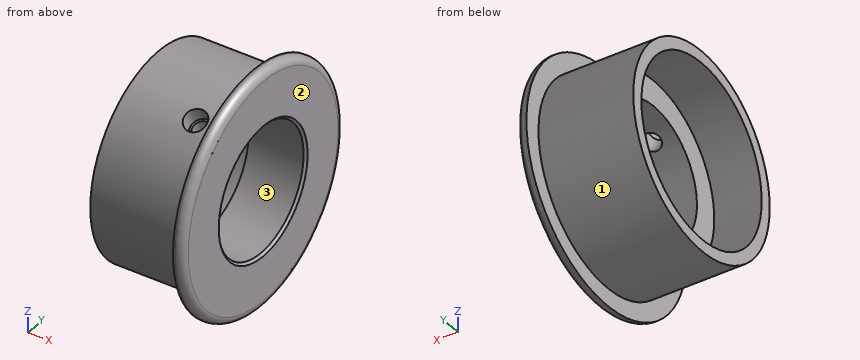
from build123d import *

# Parameters (mm, degrees)
SKETCH144_R     = 2.25
HOLE050_DEPTH   = 40.84516
SKETCH145_R     = 2.8
POCKET198_DEPTH = 4.5
CHAMFER002_SIZE = 0.6


with BuildPart() as part:
    # Sketch143 → Revolution004 (revolve)
    with BuildSketch(Plane.XZ):
        with BuildLine():
            Line((0, 25.4), (0, 29.9))
            Line((0, 29.9), (0.5, 29.9))
            ThreePointArc((2.5, 27.9), (1.914214, 29.314214), (0.5, 29.9))
            Line((2.5, 27.9), (2.5, 15.95))
            Line((2.5, 15.95), (-12, 15.95))
            Line((-12, 15.95), (-12, 22.4))
            Line((-12, 22.4), (-24, 22.4))
            Line((-24, 22.4), (-24, 25.4))
            Line((-24, 25.4), (0, 25.4))
        make_face()
    revolve(axis=Axis((0, 0, 0), (1, 0, 0)))

    # Sketch144 (on DatumPlane) → Hole050 (cut, through all)
    with BuildSketch(Plane(origin=(-6, 0, 0), x_dir=(1, 0, 0), z_dir=(0, 0.5, -0.866025))):
        Circle(SKETCH144_R)
    extrude(amount=-HOLE050_DEPTH, mode=Mode.SUBTRACT)

    # Sketch145 (on DatumPlane) → Pocket198 (cut)
    with BuildSketch(Plane(origin=(-6, -12.7, 21.997045), x_dir=(-1, 0, 0), z_dir=(0, -0.5, 0.866025))):
        Circle(SKETCH145_R)
    extrude(amount=-POCKET198_DEPTH, mode=Mode.SUBTRACT)

    # Chamfer002
    chamfer002_edges = [part.edges().sort_by_distance(p)[0] for p in [
        (2.5, 0, -15.95),
    ]]
    chamfer(chamfer002_edges, length=CHAMFER002_SIZE)


with BuildPart() as part_1:
    # Body022029 placement: moved
    add(part.part.moved(Location((194, 0, 835))))


solid = part_1.part
Model file for the job. Use its own axes, mm. Face numbers are marked on the shaded views. Give positions to 0.01 mm unless a question says otherwise; leave off trailing zeros. Order: outer loops, then holes, each group sorted by start corner. A loop starts at its lowest first (then second) coordinate and runs counter-clockwise, first axis right, second up. Notation, with made-up numbers: (86, 7) -> (92, 7) arc R28 ccw to (92, 30) -> close; hole circle Ø6 at (-14.75, 20). An arc over 180 degrees is marked (long way). Use CSV: the item, a comma, the result in double quotes.
1. Drop flat-ended pins along their axis: pin 1 (6 mm diameter, centred on x = 190, y = -12, fed in from -Z); pin 2 (8 mm diameter, centred on x = 192.5, y = -11.5, fed in from +Z); pin 3 (4 mm diameter, centred on x = 185.5, y = 16.5, fed in from +Z). Give the stop position or say it passes through.
Outcome:
pin 1,"z = 811.25"
pin 2,"z = 863.87"
pin 3,"z = 855.85"
2. Mould opens along Z. For the marked faces 1, 2 and 3 say: +Z half, -Z half, draft (parallel to the pull), parting line (faces both ways), or undercut.
Outcome:
face 1,"parting line"
face 2,"draft"
face 3,"undercut"
3. Band-saw the part on B-B, the plane y = 0. Give the cut face in (x, z).
Outcome:
outline,"(170, 809.6) -> (194, 809.6) -> (194, 805.1) -> (194.5, 805.1) arc R2 ccw to (196.5, 807.1) -> (196.5, 818.45) -> (195.9, 819.05) -> (182, 819.05) -> (182, 812.6) -> (170, 812.6) -> close; (170, 857.4) -> (182, 857.4) -> (182, 850.95) -> (195.9, 850.95) -> (196.5, 851.55) -> (196.5, 862.9) arc R2 ccw to (194.5, 864.9) -> (194, 864.9) -> (194, 860.4) -> (170, 860.4) -> close"
4. Band-saw the part on D-D, the plane x = 183.5. Give the cut face in (y, z), then the cut area to 3 significant figures.
Outcome:
outline,"circle Ø50.8 at (0, 835); hole circle Ø31.9 at (0, 835)"
area,"1,230 mm²"
5. Band-saw the part on A-A, the plane z = 835. Give the cut face in (x, y), then the cut area to 3 significant figures.
Outcome:
outline,"(170, -25.4) -> (194, -25.4) -> (194, -29.9) -> (194.5, -29.9) arc R2 ccw to (196.5, -27.9) -> (196.5, -16.55) -> (195.9, -15.95) -> (182, -15.95) -> (182, -22.4) -> (170, -22.4) -> close; (170, 22.4) -> (182, 22.4) -> (182, 15.95) -> (195.9, 15.95) -> (196.5, 16.55) -> (196.5, 27.9) arc R2 ccw to (194.5, 29.9) -> (194, 29.9) -> (194, 25.4) -> (170, 25.4) -> close"
area,"366 mm²"
6. Drill centre lines: line 1 along Y through (x, z) = (186, 834.5); line 2 along Z through (x, y) = (174.25, 0); line 3 along Z through (x, y) = (191.25, 0.5). Where is each one in solid material? Low to high. Write a range as from..to.
Outcome:
line 1,"-25.4..-15.94, 15.94..25.4"
line 2,"809.6..812.6, 857.4..860.4"
line 3,"809.6..819.06, 850.94..860.4"
7. Band-saw the part on C-C, the plane x = 175.25. Give the cut face in (y, z), then the cut area to 3 significant figures.
Outcome:
outline,"circle Ø50.8 at (0, 835); hole circle Ø44.8 at (0, 835)"
area,"451 mm²"
